CAD build for the part. Positions are in the model's coordinates, mm. A direction names the side the tool comes from. Give positions to 0.01 mm unless a question says otherwise; leave off trailing zeros. Loops run counter-clockwise (first coordinate to the right, second up) from the corner with the lowest first, then second, coordinate; pieces in that order, holes last.
```python
from build123d import *

# Parameters (mm, degrees)
BOSS_EXTRUDE9_DEPTH      = 6.35
SKETCH4_W                = 3.261538064
SKETCH4_H                = 3.965348827
CUT_EXTRUDE2_DEPTH       = 26.406776986
SKETCH5_W                = 1.630769032
SKETCH5_H                = 1.267236454
CUT_EXTRUDE6_DEPTH       = 26.406776986
SKETCH6_W                = 1.630769032
SKETCH6_H                = 1.247570224
CUT_EXTRUDE7_DEPTH       = 26.406776986
CUT_EXTRUDE9_DEPTH       = 23.902768758
CUT_EXTRUDE9_DEPTH_BACK  = 23.902768758
SKETCH8_W                = 0.566855721
SKETCH8_H                = 1.002964872
CUT_EXTRUDE10_DEPTH      = 26.406776986
CUT_EXTRUDE10_DEPTH_BACK = 26.406776986
SKETCH9_W                = 0.508
SKETCH9_H                = 1.002964872
FILLET1_R                = 0.254
FILLET2_R                = 0.254
FILLET3_R                = 0.254
FILLET4_R                = 0.508
FILLET5_R                = 0.508
SKETCH11_W               = 5.19034067
SKETCH11_H               = 2.415254944
CUT_EXTRUDE11_DEPTH      = 30.316944626
FILLET6_R                = 1.143


with BuildPart() as part:
    # Sketch2 → Boss-Extrude9 (new, symmetric)
    with BuildSketch(Plane.XY):
        with BuildLine():
            Line((-5.471488307, -10.4902), (-4.36371454, -10.4902))
            ThreePointArc((-4.36371454, -10.4902), (-3.465688928, -10.862174388), (-3.09371454, -11.7602))
            Line((-3.09371454, -11.7602), (-3.09371454, -12.937827191))
            Line((-3.09371454, -12.937827191), (-10.566399977, -12.937827191))
            Line((-10.566399977, -12.937827191), (-10.566399977, -19.301956075))
            Line((-10.566399977, -19.301956075), (10.566399977, -19.301956075))
            Line((10.566399977, -19.301956075), (10.566399977, -12.937827191))
            Line((10.566399977, -12.937827191), (3.086674887, -12.937827191))
            Line((3.086674887, -12.937827191), (3.086674887, -11.7602))
            ThreePointArc((3.086674887, -11.7602), (3.458649275, -10.862174388), (4.356674887, -10.4902))
            Line((4.356674887, -10.4902), (5.476039751, -10.4902))
            Line((5.476039751, -10.4902), (5.476039751, -7.173536635))
            Line((5.476039751, -7.173536635), (3.650231899, -5.31386943))
            ThreePointArc((3.650231899, -5.31386943), (3.496357897, -5.285953607), (3.418648834, -5.421665813))
            ThreePointArc((3.418648834, -5.421665813), (0.00035136, -9.18188013), (-3.418715481, -5.422365367))
            ThreePointArc((-3.418715481, -5.422365367), (-3.496506609, -5.286643819), (-3.650404442, -5.314701882))
            Line((-3.650404442, -5.314701882), (-5.471488307, -7.173600332))
            Line((-5.471488307, -7.173600332), (-5.471488307, -10.4902))
        make_face()
    extrude(amount=BOSS_EXTRUDE9_DEPTH, both=True)

    # Sketch4 → Cut-Extrude2 (cut, through all)
    with BuildSketch(Plane.XY.offset(6.35)):
        with Locations((0, -11.95811765)):
            Rectangle(SKETCH4_W, SKETCH4_H)
    extrude(amount=-CUT_EXTRUDE2_DEPTH, mode=Mode.SUBTRACT)

    # Sketch5 → Cut-Extrude6 (cut, through all)
    with BuildSketch(Plane.XY.offset(6.35)):
        with Locations((-0.815384516, -9.341825009)):
            Rectangle(SKETCH5_W, SKETCH5_H)
    extrude(amount=-CUT_EXTRUDE6_DEPTH, mode=Mode.SUBTRACT)

    # Sketch6 → Cut-Extrude7 (cut, through all)
    with BuildSketch(Plane(origin=(0, 0, -6.35), x_dir=(-1, 0, 0), z_dir=(0, 0, -1))):
        with Locations((-0.815384516, -9.351658124)):
            Rectangle(SKETCH6_W, SKETCH6_H)
    extrude(amount=-CUT_EXTRUDE7_DEPTH, mode=Mode.SUBTRACT)

    # Sketch8 → Cut-Extrude9 (cut, two sides: drawn at the far end of the back side and taken through both)
    with BuildSketch(Plane.XY.offset(-CUT_EXTRUDE9_DEPTH_BACK)):
        with Locations((-3.377142401, -13.439309627)):
            Rectangle(SKETCH8_W, SKETCH8_H)
    extrude(amount=CUT_EXTRUDE9_DEPTH + CUT_EXTRUDE9_DEPTH_BACK, mode=Mode.SUBTRACT)

    # Sketch9 → Cut-Extrude10 (cut, two sides: drawn at the far end of the back side and taken through both)
    with BuildSketch(Plane.XY.offset(6.35).offset(-CUT_EXTRUDE10_DEPTH_BACK)):
        with Locations((3.340674887, -13.439309627)):
            Rectangle(SKETCH9_W, SKETCH9_H)
    extrude(amount=CUT_EXTRUDE10_DEPTH + CUT_EXTRUDE10_DEPTH_BACK, mode=Mode.SUBTRACT)

    # Fillet1
    fillet1_edges = [part.edges().sort_by_distance(p)[0] for p in [
        (-3.09371454, -13.940792063, 0),
    ]]
    fillet(fillet1_edges, radius=FILLET1_R)

    # Fillet2
    fillet2_edges = [part.edges().sort_by_distance(p)[0] for p in [
        (-3.660570261, -13.940792063, 0),
    ]]
    fillet(fillet2_edges, radius=FILLET2_R)

    # Fillet3
    fillet3_edges = [part.edges().sort_by_distance(p)[0] for p in [
        (3.594674887, -13.940792063, 0),
        (3.086674887, -13.940792063, 0),
        (1.630769032, -13.940792063, 0),
        (-1.630769032, -13.940792063, 0),
    ]]
    fillet(fillet3_edges, radius=FILLET3_R - 0.0001)  # a hair under: the kernel refuses the full size

    # Fillet4
    fillet4_edges = [part.edges().sort_by_distance(p)[0] for p in [
        (-10.566399977, -12.937827191, 0),
    ]]
    fillet(fillet4_edges, radius=FILLET4_R)

    # Fillet5
    fillet5_edges = [part.edges().sort_by_distance(p)[0] for p in [
        (-10.566399977, -19.301956075, 0),
        (10.566399977, -12.937827191, 0),
        (10.566399977, -19.301956075, 0),
    ]]
    fillet(fillet5_edges, radius=FILLET5_R)

    # Sketch11 → Cut-Extrude11 (cut, through all)
    with BuildSketch(Plane.ZY.offset(10.566399977)):
        with Locations((0, -16.044100378)):
            Rectangle(SKETCH11_W, SKETCH11_H)
    extrude(amount=-CUT_EXTRUDE11_DEPTH, mode=Mode.SUBTRACT)

    # Fillet6
    fillet6_edges = [part.edges().sort_by_distance(p)[0] for p in [
        (0, -14.836472906, 2.595170335),
        (0, -17.25172785, 2.595170335),
        (0, -17.25172785, -2.595170335),
        (0, -14.836472906, -2.595170335),
    ]]
    fillet(fillet6_edges, radius=FILLET6_R)


solid = part.part
```
1. Probe line 1 along X through (y, z) = (-13.5, 1.25); line 2 along X through (y, z) = (-9.75, 2); line 3 along Y through (x, z) = (7.75, -3.25). List the from-to ranges inside material, lowest first.
Responses:
line 1: x = -10.57 to -3.66, -3.09 to -1.63, 1.63 to 3.09, 3.59 to 10.57
line 2: x = -5.47 to -1.63, 1.63 to 5.48
line 3: y = -19.3 to -12.94
2. Saw through at C-C, the plane y = -15.25. List the corners of the cut face in (x, z), and give its area (3 significant figures).
Responses:
outline: (-10.57, -6.35) - (10.57, -6.35) - (10.57, -2.33) - (-10.57, -2.33) - close; (-10.57, 2.33) - (10.57, 2.33) - (10.57, 6.35) - (-10.57, 6.35) - close
area: 170 mm2
3. Saw through at A-A, the plane x = 8.5. List the corners of the cut face in (y, z), and give its area (3 significant figures).
Responses:
outline: (-19.3, -6.35) - (-12.94, -6.35) - (-12.94, 6.35) - (-19.3, 6.35) - close; hole (-17.25, -1.45) arc R1.14 ccw to (-16.11, -2.6) - (-15.98, -2.6) arc R1.14 ccw to (-14.84, -1.45) - (-14.84, 1.45) arc R1.14 ccw to (-15.98, 2.6) - (-16.11, 2.6) arc R1.14 ccw to (-17.25, 1.45) - close
area: 69.4 mm2
4. Saw through at B-B, the plane y = -6.5. List the corners of the cut face in (x, z).
Responses:
outline: (-4.81, -6.35) - (-3.35, -6.35) - (-3.35, 6.35) - (-4.81, 6.35) - close; (3.35, -6.35) - (4.81, -6.35) - (4.81, 6.35) - (3.35, 6.35) - close
5. Drop flat-ended pins along their axis: pin 1 (4 mm diameter, centred on y = -10.5, z = 1.5, fed in from +X); pin 2 (1.9 mm diameter, centred on x = -7, z = 1.5, fed in from +Y); pin 3 (3.5 mm diameter, centred on y = -8.5, z = -1.5, fed in from -X). Give the stop position or say it passes through.
Responses:
pin 1: stops at x = 5.48
pin 2: stops at y = -12.94
pin 3: stops at x = -5.47
6. Tool access for faces 5 (the face through (0, -14.836, 0)), 6 (the face through (3.087, -13, 0)), 7 (the face through (0, -13.941, 0)): list every direction of +Z, -Z, +X, -X, +Y, -Y with a clear straight run to the whole face (end or side of a thin tool).
Responses:
face 5: +X, -X
face 6: +Z, -Z
face 7: +Z, -Z, +Y
7. Pull direction Y, two halves, no side cores. Call faces 1 (the face through (-4.548, -6.231, 0.089)), 2 (the face through (3.45, -10.87, 0.09)), 3 (the face through (5.476, -9, 0)), 4 (the face through (0, -19.302, 0)): released by +Y, released by -Y, zero draft, split by the parting line, or undercut.
Responses:
face 1: released by +Y
face 2: undercut
face 3: zero draft
face 4: released by -Y
